from build123d import *

# Parameters (mm, degrees)
SKETCH1_W           = 20
SKETCH1_H           = 80
BOSS_EXTRUDE1_DEPTH = 40
BOSS_EXTRUDE2_DEPTH = 80
CUT_EXTRUDE2_DEPTH  = 40
CUT_EXTRUDE4_DEPTH  = 81


with BuildPart() as part:
    # Sketch1 → Boss-Extrude1 (new body, symmetric)
    with BuildSketch(Plane.XY):
        with Locations((10, 40)):
            Rectangle(SKETCH1_W, SKETCH1_H)
    extrude(amount=BOSS_EXTRUDE1_DEPTH, both=True)

    # Sketch2 → Boss-Extrude2 (add)
    with BuildSketch(Plane(origin=(0, 0, 0), x_dir=(0, 0, -1), z_dir=(1, 0, 0))):
        with BuildLine():
            Line((40, 80), (20, 80))
            Line((20, 80), (-40, 20))
            Line((-40, 20), (-40, 0))
            Line((-40, 0), (0, 0))
            ThreePointArc((0, 0), (11.715728753, 28.284271247), (40, 40))
            Line((40, 40), (40, 80))
        make_face()
    extrude(amount=BOSS_EXTRUDE2_DEPTH)

    # Sketch4 → Cut-Extrude2 (cut)
    with BuildSketch(Plane(origin=(80, 0, 0), x_dir=(0, 0, -1), z_dir=(1, 0, 0))):
        Polygon((0, 60), (0, 40), (-20, 40), align=None)
    extrude(amount=-CUT_EXTRUDE2_DEPTH, mode=Mode.SUBTRACT)

    # Sketch5 → Cut-Extrude4 (cut, through all)
    with BuildSketch(Plane(origin=(0, 0, 0), x_dir=(1, 0, 0), z_dir=(0, 1, 0))):
        with BuildLine():
            Line((40, 40), (50, 40))
            ThreePointArc((50, 40), (40, 30), (30, 40))
            Line((30, 40), (40, 40))
        make_face()
    extrude(amount=CUT_EXTRUDE4_DEPTH, mode=Mode.SUBTRACT)


solid = part.part
Could you check a few things on this model? Use its own coordinates, in mm. A direction names the side the tool comes from. Coordinates: 2 decimals unless noted, no trailing zeros. Order: outer loops, then holes, each group sorted by start corner. A loop starts at its lowest first (then second) coordinate and runs counter-clockwise, first axis right, second up. Notation, with made-up numbers: (-20, -1.75) -> (12, -1.75) arc R26 cw to (12, 25.25) -> close; hole circle Ø9 at (87, 11). An arc over 180 degrees is marked (long way). One line per question, with ' | ' between items.
Q1. Imagine slicing it at B-B on x = 21.5. Please give me the cut outline in (y, z).
Return value:
outline: (0, 0) arc R40 cw to (40, -40) -> (80, -40) -> (80, -20) -> (20, 40) -> (0, 40) -> close
Q2. Imagine slicing it at A-A on y = 54.5. Please give me the cut outline in (x, z).
Return value:
outline: (0, -40) -> (30, -40) arc R10 cw to (50, -40) -> (80, -40) -> (80, 0) -> (40, 0) -> (40, 5.5) -> (20, 5.5) -> (20, 40) -> (0, 40) -> close
Q3. If I drill on L1, parallel to X at y = 32.5, z = -28; L2, parallel to Z at x = 71, y = 43; L3, parallel to X at y = 46.5, z = -34, over which ranges is the centre line in solid material (lowest first)?
Return value:
L1: 0 to 20 | L2: -40 to 0 | L3: 0 to 32, 48 to 80
Q4. Thinking about a two-plate mould opening in X: for faces 1 (the face through (40, 59, -30)), 2 (the face through (0, 39, 1)), 3 (the face through (80, 41, -8)), which applies, pulls with the +X half, pulls with the -X half, needs draft (parallel to the pull), parting line crosses it, or undercut?
Return value:
face 1: undercut | face 2: pulls with the -X half | face 3: pulls with the +X half
Q5. I'm going to push flat-ended pins straight in: P1, Ø6, axis at x = 72, y = 72, coming from the +Z side; P2, Ø5, axis at x = 62.5, z = 31, coming from the +Y side; P3, Ø2, axis at x = 66.5, z = -22, coming from the -Y side. Where does each tip first touch, or does it pass through?
Return value:
P1: z = -9 | P2: y = 31.5 | P3: y = 35.2
Q6. Imagine slicing it at D-D on y = 43. Please give me the cut outline in (x, z).
Return value:
outline: (0, -40) -> (30, -40) arc R10 cw to (50, -40) -> (80, -40) -> (80, 0) -> (40, 0) -> (40, 17) -> (20, 17) -> (20, 40) -> (0, 40) -> close
Q7. Imagine slicing it at C-C on z = 12. Please give me the cut outline in (x, y).
Return value:
outline: (0, 0) -> (80, 0) -> (80, 40) -> (40, 40) -> (40, 48) -> (20, 48) -> (20, 80) -> (0, 80) -> close
Q8. On a 3-axis mill with a long thin cutter (end or side, diameter ignored), from which of +Z, -Z, +X, -X, +Y, -Y can I reach the whole of each face in a straight line? I mean faces 4 (the face through (65, 60, -40)), 5 (the face through (49.58, 27.972, -11.406)), 6 (the face through (60, 50, 0)). Say none if no direction works.
Return value:
face 4: -Z, +X, -X, +Y, -Y | face 5: -Z, +X, -Y | face 6: +Z, +X, +Y
